Check sheet for the modelled part. Datum: model origin and axes. Units: mm. A direction names the side the tool comes from. Give positions to 0.01 mm unless a question says otherwise; leave off trailing zeros. Write each loop counter-clockwise with the first axis right and the second up, starting at its lowest first coordinate (ties: lowest second). Pieces come first, ordered by that corner, then holes. Notation, with made-up numbers: (89, 17) -> (123, 17) arc R18 ccw to (123, 50) -> close; hole circle Ø8 at (23.5, 27). An arc over 180 degrees is marked (long way). Use a Markdown table: item, result. Add a question column.
1. Gauge pin test, flat ends, axial feed: P1, Ø1, axis at y = 2.5, z = -2, coming from the -X side; P2, Ø1.9, axis at x = 0, z = 0, coming from the +Y side; P3, Ø3.5, axis at x = -4.24, z = -4.24, coming from the -Y side; P4, Ø0.9, axis at y = 1, z = 13.5, coming from the -X side. Record the tip position at first contact, or that the pin passes through.
2. Release check for a two-part mould opening along Z. For faces 1 (the cylindrical face through (-5.5, 1.5, 14)), 2 (the cylindrical face through (-0.07, 1.48, 11.6)), 3 (the cylindrical face through (12, 2, -6)), 4 (the cylindrical face through (11.56, 1.52, 0.35)) record: released by +Z, released by -Z, zero draft, split by the parting line, or undercut.
3. Cross-section at C-C (x = 9). Enter the section's corners in (y, z), then the cut area to 3 significant figures.
4. Set-up check for faces 5 (the flat face through (-7, 1, -15)), 6 (the flat face through (7, 1, 15)), 7 (the flat face through (-7, 1, 15)): record each of +Z, -Z, +X, -X, +Y, -Y from which the full face is reachable in a straight line by a thin tool's end or side.
5. Cross-section at A-A (z = 0). Enter the section's corners in (x, y), then the cut area to 3 significant figures.
6. Scan lines: probe 1 along X at (y, z) = (1.25, 10); probe 2 along Z at (x, y) = (-1, 2.75); probe 3 along X at (y, z) = (2.05, 0). Record each from-to range of solid material in increasing order. Write a range as [from, to].
7. Cross-section at B-B (x = 0). Enter the section's corners in (y, z).
8. Cross-section at D-D (y = 2.4). Count the separate pieces of the cut face and the enclosed holes in it, then the cut area to 3 significant figures.
from build123d import *

# Parameters (mm, degrees)
SKETCH_1_W                = 16
SKETCH_1_H                = 30
SKETCH_1_R                = 1.6
EXTRUDE_1_DEPTH           = 3
SKETCH_2_W                = 9
SKETCH_2_H                = 3
EXTRUDE_2_DEPTH           = 3
SKETCH_3_R                = 1
CUT_EXTRUDE_1_DEPTH       = 20.924858845
SKETCH_4_R                = 1.6
EXTRUDE_3_DEPTH           = 3
SKETCH_8_R                = 1
CUT_EXTRUDE_3_DEPTH       = 24
FILLET_1_R                = 3
HOLE_WIZARD_1_D           = 2.2
HOLE_WIZARD_1_CSINK_D     = 4.5
HOLE_WIZARD_1_CSINK_ANGLE = 90


with BuildPart() as part:
    # 草图1 → 凸台-拉伸1 (new body)
    with BuildSketch(Plane(origin=(0, 0, 0), x_dir=(1, 0, 0), z_dir=(0, 1, 0))):
        Rectangle(SKETCH_1_W, SKETCH_1_H)
        with Locations(Location((0, 0, 0), (0, 0, 270))):
            Circle(SKETCH_1_R, mode=Mode.SUBTRACT)
        with Locations(Location((0, 10, 0), (0, 0, 270))):
            Circle(SKETCH_1_R, mode=Mode.SUBTRACT)
        with Locations(Location((0, -10, 0), (0, 0, 90))):
            Circle(SKETCH_1_R, mode=Mode.SUBTRACT)
    extrude(amount=EXTRUDE_1_DEPTH)

    # 草图2 → 凸台-拉伸2 (add)
    with BuildSketch(Plane(origin=(0, 3, 0), x_dir=(1, 0, 0), z_dir=(0, 1, 0))):
        with Locations((0, 16.5)):
            Rectangle(SKETCH_2_W, SKETCH_2_H)
        with Locations((0, -16.5)):
            Rectangle(SKETCH_2_W, SKETCH_2_H)
    extrude(amount=-EXTRUDE_2_DEPTH)

    # 草图3 → 切除-拉伸1 (cut, through all)
    with BuildSketch(Plane(origin=(0, 3, 0), x_dir=(1, 0, 0), z_dir=(0, 1, 0))):
        with Locations((-5.5, 15)):
            Circle(SKETCH_3_R)
        with Locations((5.5, 15)):
            Circle(SKETCH_3_R)
        with Locations((5.5, -15)):
            Circle(SKETCH_3_R)
        with Locations((-5.5, -15)):
            Circle(SKETCH_3_R)
    extrude(amount=-CUT_EXTRUDE_1_DEPTH, mode=Mode.SUBTRACT)

    # 草图4 → 凸台-拉伸3 (add)
    # profile 1 of 2: a face of its own
    with BuildSketch(Plane(origin=(0, 3, 0), x_dir=(1, 0, 0), z_dir=(0, 1, 0))):
        with BuildLine():
            Line((8, -7.6), (8, 7.6))
            ThreePointArc((8, 7.6), (11.623231276, 6.329039095), (13.658536585, 3.073170732))
            ThreePointArc((13.658536585, 3.073170732), (14, 0), (13.658536585, -3.073170732))
            ThreePointArc((13.658536585, -3.073170732), (11.623231276, -6.329039095), (8, -7.6))
        make_face()
        with Locations(Location((10, 0, 0), (0, 0, 90))):
            Circle(SKETCH_4_R, mode=Mode.SUBTRACT)
    # profile 2 of 2: a face of its own
    with BuildSketch(Plane(origin=(0, 3, 0), x_dir=(1, 0, 0), z_dir=(0, 1, 0))):
        with BuildLine():
            Line((-8, 7.6), (-8, -7.6))
            ThreePointArc((-8, -7.6), (-11.623231276, -6.329039095), (-13.658536585, -3.073170732))
            ThreePointArc((-13.658536585, -3.073170732), (-14, 0), (-13.658536585, 3.073170732))
            ThreePointArc((-13.658536585, 3.073170732), (-11.623231276, 6.329039095), (-8, 7.6))
        make_face()
        with Locations(Location((-10, 0, 0), (0, 0, 270))):
            Circle(SKETCH_4_R, mode=Mode.SUBTRACT)
    extrude(amount=-EXTRUDE_3_DEPTH)

    # 草图8 → 切除-拉伸3 (cut, through all)
    with BuildSketch(Plane(origin=(0, 3, 0), x_dir=(1, 0, 0), z_dir=(0, 1, 0))):
        with Locations(Location((-4.242640687, 4.242640687, 0), (0, 0, 270))):
            Circle(SKETCH_8_R)
        with Locations(Location((4.242640687, 4.242640687, 0), (0, 0, 270))):
            Circle(SKETCH_8_R)
        with Locations(Location((4.242640687, -4.242640687, 0), (0, 0, 270))):
            Circle(SKETCH_8_R)
        with Locations(Location((-4.242640687, -4.242640687, 0), (0, 0, 270))):
            Circle(SKETCH_8_R)
    extrude(amount=-CUT_EXTRUDE_3_DEPTH, mode=Mode.SUBTRACT)

    # 圆角1
    fillet_1_edges = [part.edges().sort_by_distance(p)[0] for p in [
        (-8, 1.5, 7.6),
        (-8, 1.5, -7.6),
        (8, 1.5, 7.6),
        (8, 1.5, -7.6),
    ]]
    fillet(fillet_1_edges, radius=FILLET_1_R)

    # 打孔尺寸(%根据十字)槽沉头木螺钉的类型1 (through all)
    with Locations(Plane.XZ):
        with Locations((-4.242640687, -4.242640687), (4.242640687, -4.242640687), (-4.242640687, 4.242640687), (4.242640687, 4.242640687)):
            CounterSinkHole(HOLE_WIZARD_1_D / 2, HOLE_WIZARD_1_CSINK_D / 2, counter_sink_angle=HOLE_WIZARD_1_CSINK_ANGLE)


solid = part.part
Worked answers:
| question | item | result |
|---|---|---|
| 1 | P1 | stops at x = -13.92 |
| 1 | P2 | passes through |
| 1 | P3 | stops at y = 0.5 |
| 1 | P4 | stops at x = -8 |
| 2 | face 1 | released by +Z |
| 2 | face 2 | undercut |
| 2 | face 3 | released by -Z |
| 2 | face 4 | undercut |
| 3 | outline | (0, -7.84) -> (3, -7.84) -> (3, -1.25) -> (0, -1.25) -> close; (0, 1.25) -> (3, 1.25) -> (3, 7.84) -> (0, 7.84) -> close |
| 3 | area | 39.5 mm² |
| 4 | face 5 | -Z, -X, +Y, -Y |
| 4 | face 6 | +Z, +X, +Y, -Y |
| 4 | face 7 | +Z, -X, +Y, -Y |
| 5 | outline | (-14, 0) -> (-11.6, 0) -> (-11.6, 3) -> (-14, 3) -> close; (-8.4, 0) -> (-1.6, 0) -> (-1.6, 3) -> (-8.4, 3) -> close; (1.6, 0) -> (8.4, 0) -> (8.4, 3) -> (1.6, 3) -> close; (11.6, 0) -> (14, 0) -> (14, 3) -> (11.6, 3) -> close |
| 5 | area | 55.2 mm² |
| 6 | probe 1 | x = [-8, -1.6], [1.6, 8] |
| 6 | probe 2 | z = [-18, -11.25], [-8.75, -1.25], [1.25, 8.75], [11.25, 18] |
| 6 | probe 3 | x = [-14, -11.6], [-8.4, -1.6], [1.6, 8.4], [11.6, 14] |
| 7 | outline | (0, -18) -> (3, -18) -> (3, -11.6) -> (0, -11.6) -> close; (0, -8.4) -> (3, -8.4) -> (3, -1.6) -> (0, -1.6) -> close; (0, 1.6) -> (3, 1.6) -> (3, 8.4) -> (0, 8.4) -> close; (0, 11.6) -> (3, 11.6) -> (3, 18) -> (0, 18) -> close |
| 8 | separate pieces | 1 |
| 8 | enclosed holes | 9 |
| 8 | area | 625 mm² |
